```python
from build123d import *

# Parameters (mm, degrees)
EXTRU_MINCE1_DEPTH      = 27.5
CONG_2_R                = 2
ESQUISSE2_R             = 1.6
ENL_V_MAT_EXTRU_1_DEPTH = 33.314857264
ESQUISSE3_R             = 1.6
ENL_V_MAT_EXTRU_2_DEPTH = 33.314857386
ENL_V_START             = -3
ENL_V_MAT_EXTRU_3_DEPTH = 30.314857423
ENL_V_MAT_EXTRU_4_DEPTH = 30.314857386
CONG_1_R                = 2


with BuildPart() as part:
    # Esquisse1 → Extru.-Mince1 (new, symmetric)
    with BuildSketch(Plane(origin=(0, 0, 0), x_dir=(0, 0, -1), z_dir=(1, 0, 0))):
        Polygon((12, 0), (0, 0), (0, -12), (6, -12), (6, -6), (12, -6), align=None)
    extrude(amount=EXTRU_MINCE1_DEPTH, both=True)

    # Cong_2
    cong_2_edges = [part.edges().sort_by_distance(p)[0] for p in [
        (0, -6, -12),
        (0, -6, -6),
        (0, -12, -6),
    ]]
    fillet(cong_2_edges, radius=CONG_2_R)

    # Esquisse2 → Enl_v. mat.-Extru.1 (cut, through all)
    with BuildSketch(Plane(origin=(0, 0, 0), x_dir=(1, 0, 0), z_dir=(0, 1, 0))):
        with Locations(Location((-17, 7.5, 0), (0, 0, 270))):
            Circle(ESQUISSE2_R)
        with Locations(Location((17, 7.5, 0), (0, 0, 290.364128873))):
            Circle(ESQUISSE2_R)
    extrude(amount=-ENL_V_MAT_EXTRU_1_DEPTH, mode=Mode.SUBTRACT)

    # Esquisse3 → Enl_v. mat.-Extru.2 (cut, through all)
    with BuildSketch(Plane.XY):
        with Locations((22.5, -7.5)):
            Circle(ESQUISSE3_R)
        with Locations(Location((-22.5, -7.5, 0), (0, 0, 341.790043136))):
            Circle(ESQUISSE3_R)
    extrude(amount=-ENL_V_MAT_EXTRU_2_DEPTH, mode=Mode.SUBTRACT)

    # Esquisse4 → Enl_v. mat.-Extru.3 (cut, through all)
    with BuildSketch(Plane(origin=(0, 0, 0), x_dir=(1, 0, 0), z_dir=(0, 1, 0)).offset(ENL_V_START)):
        Polygon((-14.25, 9.08771324), (-17, 10.675426481), (-19.75, 9.08771324), (-19.75, 5.91228676), (-17, 4.324573519), (-14.25, 5.91228676), align=None)
        Polygon((19.75, 9.08771324), (17, 10.675426481), (14.25, 9.08771324), (14.25, 5.91228676), (17, 4.324573519), (19.75, 5.91228676), align=None)
    extrude(amount=-ENL_V_MAT_EXTRU_3_DEPTH, mode=Mode.SUBTRACT)

    # Esquisse5 → Enl_v. mat.-Extru.4 (cut, through all)
    with BuildSketch(Plane.XY.offset(ENL_V_START)):
        Polygon((25.25, -5.91228676), (22.5, -4.324573519), (19.75, -5.91228676), (19.75, -9.08771324), (22.5, -10.675426481), (25.25, -9.08771324), align=None)
        Polygon((-19.75, -9.08771324), (-19.75, -5.91228676), (-22.5, -4.324573519), (-25.25, -5.91228676), (-25.25, -9.08771324), (-22.5, -10.675426481), align=None)
    extrude(amount=-ENL_V_MAT_EXTRU_4_DEPTH, mode=Mode.SUBTRACT)

    # Cong_1
    cong_1_edges = [part.edges().sort_by_distance(p)[0] for p in [
        (27.5, -2, -12),
        (-27.5, -9, -6),
        (27.5, -9, -6),
        (-27.5, -6, -9),
        (-27.5, -12, -2),
        (-27.5, -5.414213562, -11.414213562),
        (-27.5, -11.414213562, -5.414213562),
        (27.5, -12, -2),
        (27.5, -6, -9),
        (27.5, -5.414213562, -11.414213562),
        (27.5, -11.414213562, -5.414213562),
        (-27.5, -6.585786438, -6.585786438),
        (27.5, -6.585786438, -6.585786438),
        (-27.5, -2, -12),
    ]]
    fillet(cong_1_edges, radius=CONG_1_R)


solid = part.part
```
For this review, take the finished solid that the model builds, in its own axes (mm). A direction names the side the tool comes from. Coordinates: 2 decimals unless noted, no trailing zeros. Write each loop counter-clockwise with the first axis right and the second up, starting at its lowest first coordinate (ties: lowest second). Pieces come first, ordered by that corner, then holes. Notation, with made-up numbers: (-25.5, 74) - (-3.5, 74) arc R16 ccw to (-3.5, 97) - close; hole circle Ø2 at (-34, -20). An arc over 180 degrees is marked (long way). Answer in a Markdown table with one row per item. Add a question column.
Q1. We need section D-D, the plane z = -5.25. Count the separate pieces of the cut face and the enclosed holes in it, and give its area (3 significant figures).
Q2. For P1, Ø6, axis at x = -12.5, y = -10, coming from the -Z side; P2, Ø6, axis at x = 22.5, y = -8, coming from the -Z side; P3, Ø3, axis at x = -18, z = -7, coming from the -Y side; P4, Ø1.9, axis at x = 22.5, y = -7.5, coming from the -Z side, all flat-tipped, find the tip position at first contact; note any pin that passes through.
Q3. We need section C-C, the plane y = -1.75. State the section outline as (x, z) points.
Q4. For probe 1 along X at (y, z) = (-0.85, -7.5); probe 2 along X at (y, z) = (-9.75, -3.25); probe 3 along Z at (x, y) = (20, -7), list the stretches that pass through material, from the lowest coordinate up.
Q5. Tool access review of faces 4 (the cylindrical face through (-15.92, -1.48, -8.68)), 5 (the flat face through (-15.606, -4.479, -9.87)), 6 (the flat face through (-20.4, -9.7, -6)), 7 (the flat face through (-27.5, -4, -4)), 8 (the flat face through (23.894, -5.13, -7.424)): name each direction out of +Z, -Z, +X, -X, +Y, -Y from which nothing blocks a thin tool from reaching the whole face with its end or side.
Q6. Draft analysis for pull direction Y (two halves, no side actions). For faces 1 (the flat face through (-25.1, -9.4, -6)), 2 (the cylindrical face through (-26.93, -5.4, -9.01)), 3 (the flat face through (25.25, -8, -5)), state which applies: +Y half, -Y half, draft (parallel to the pull), parting line (faces both ways), or undercut.
Q7. We need section B-B, the plane x = -13.5. State the section outline as (y, z) points.
Q8. We need section A-A, the plane y = -8.5. State the section outline as (x, z) points, and give its area (3 significant figures).
Answer list:
| question | item | result |
|---|---|---|
| 1 | separate pieces | 1 |
| 1 | enclosed holes | 2 |
| 1 | area | 523 mm2 |
| 2 | P1 | stops at z = -6.27 |
| 2 | P2 | stops at z = -6.4 |
| 2 | P3 | stops at y = -3 |
| 2 | P4 | passes through |
| 3 | outline | (-27.5, -10) arc R2 ccw to (-25.5, -12) - (25.5, -12) arc R2 ccw to (27.5, -10) - (27.5, 0) - (-27.5, 0) - close; hole circle Ø3.2 at (-17, -7.5); hole circle Ø3.2 at (17, -7.5) |
| 4 | probe 1 | x = -27.5 to -18.6, -15.4 to 15.4, 18.6 to 27.5 |
| 4 | probe 2 | x = -27.5 to -24.1, -20.9 to 20.9, 24.1 to 27.5 |
| 4 | probe 3 | z = -3 to 0 |
| 5 | face 4 | +Y, -Y |
| 5 | face 5 | -Y |
| 5 | face 6 | -Z, +X, -X, -Y |
| 5 | face 7 | +Z, -Z, -X, +Y, -Y |
| 5 | face 8 | -Z |
| 6 | face 1 | draft |
| 6 | face 2 | -Y half |
| 6 | face 3 | undercut |
| 7 | outline | (-12, -4) arc R2 ccw to (-10, -6) - (-8, -6) arc R2 cw to (-6, -8) - (-6, -10) arc R2 ccw to (-4, -12) - (0, -12) - (0, 0) - (-12, 0) - close |
| 8 | outline | (-27.5, -4) arc R2 ccw to (-25.5, -6) - (-25.25, -6) - (-25.25, -3) - (-23.75, -3) - (-23.75, 0) - (-27.5, 0) - close; (-21.25, -3) - (-19.75, -3) - (-19.75, -5.91) - (-17, -4.32) - (-14.25, -5.91) - (-14.25, -6) - (14.25, -6) - (14.25, -5.91) - (17, -4.32) - (19.75, -5.91) - (19.75, -3) - (21.25, -3) - (21.25, 0) - (-21.25, 0) - close; (23.75, -3) - (25.25, -3) - (25.25, -6) - (25.5, -6) arc R2 ccw to (27.5, -4) - (27.5, 0) - (23.75, 0) - close |
| 8 | area | 271 mm2 |
